Autodesk Fusion 360 part; units mm, degrees
sketch "Sketch1" plane through (0, 0, 0) normal (0, 0, 1) x (1, 0, 0)
  line L0 (50, 50) -> (-50, 50)
  line L1 (-50, 50) -> (-50, -50)
  line L2 (-50, -50) -> (50, -50)
  line L3 (50, -50) -> (50, 50)
  line L4 (50, 50) -> (-50, -50) construction
  line L5 (-50, 50) -> (50, -50) construction
  line L6 (40, -40) -> (-40, -40)
  line L7 (-40, -40) -> (-40, 40)
  line L8 (-40, 40) -> (40, 40)
  line L9 (40, 40) -> (40, -40)
  line L10 (40, -40) -> (-40, 40) construction
  line L11 (-40, -40) -> (40, 40) construction
  dimension "d1" = 100
  dimension "d2" = 100
  dimension "d3" = 80
  dimension "d4" = 80
extrude "Extrude1" add sketch "Sketch1" along normal blind 10
sketch "Sketch2" plane through (0, -40, 0) normal (0, 1, 0) x (-1, 0, 0)
  line L0 (-40, 0) -> (40, 0)
  line L1 (40, 0) -> (40, 10)
  line L2 (40, 10) -> (-40, 10)
  line L3 (-40, 10) -> (-40, 0)
  line L4 (0, 10) -> (0, 0) construction
  line L5 (-40, 5) -> (40, 5) construction
  line L6 (43, 3.5) -> (-43, 3.5)
  line L7 (-43, 3.5) -> (-43, 6.5)
  line L8 (-43, 6.5) -> (43, 6.5)
  line L9 (43, 6.5) -> (43, 3.5)
  line L10 (43, 3.5) -> (-43, 6.5) construction
  line L11 (-43, 3.5) -> (43, 6.5) construction
  point P0 (0, 5)
  dimension "d9" = 86
  dimension "d10" = 3
extrude "Extrude2" cut sketch "Sketch2" along normal blind 85 and the other way blind 5 contours L1 L3 L6 L8
extrude "Extrude3" cut sketch "Sketch2" along normal blind 80 contours L3 L6 L7 L8 | L1 L6 L8 L9
sketch "Sketch3" plane through (0, 0, 10) normal (0, 0, 1) x (-1, 0, 0)
  line L0 (40, -40) -> (-40, -40)
  line L1 (-40, -40) -> (-40, 40)
  line L2 (-40, 40) -> (40, 40)
  line L3 (40, 40) -> (40, -40)
  line L4 (-50, 50) -> (-50, -50)
  line L5 (-50, -50) -> (50, -50)
  line L6 (50, -50) -> (50, 50)
  line L7 (50, 50) -> (-50, 50)
  line L8 (40, -40) -> (40, -50) construction
  line L9 (40, -40) -> (50, -40) construction
  line L10 (45, -40) -> (45, -50) construction
  line L11 (40, -45) -> (50, -45) construction
  circle A0 centre (45, -45) radius 2.5
  circle A1 centre (45, 45) radius 2.5
  dimension "d17" = 5
  dimension "d20" = -90
  dimension "d21" = 90
extrude "Extrude4" cut sketch "Sketch3" against normal blind 3 contours A0 | A1
sketch "Sketch4" plane through (50, 0, 0) normal (1, 0, 0) x (0, 1, 0)
  line L0 (-50, 0) -> (50, 0)
  line L1 (50, 0) -> (50, 10)
  line L2 (50, 10) -> (-50, 10)
  line L3 (-50, 10) -> (-50, 0)
  line L4 (-40, 3.5) -> (-40, 6.5)
  line L5 (-40, 5) -> (-50, 5) construction
  circle A0 centre (-45, 5) radius 2.5
  circle A1 centre (0, 5) radius 2.5
  circle A2 centre (45, 5) radius 2.5
  dimension "d24" = 5
  dimension "d27" = 90
  dimension "d28" = 0
extrude "Extrude5" cut sketch "Sketch4" against normal blind 3 contours A0 | A2
equation "d9 = 80 mm + 6 mm"
equation "d30 = f8e7f7a2-a6e5-415b-bf69-f4a3084041c5"
Source: CAD feature listing. Evaluate the final solid. Frame: model axes, mm. A direction names the side the tool comes from. Give positions to 0.01 mm unless a question says otherwise; leave off trailing zeros. Write each loop counter-clockwise with the first axis right and the second up, starting at its lowest first coordinate (ties: lowest second). Pieces come first, ordered by that corner, then holes. Notation, with made-up numbers: M 39,71 L 52,71 A23 cw 52,96 Z; hole C 47,83.25 d7. An arc over 180 degrees is marked long. Return JSON: item names as keys, results as strings. Group by question number.
1) Cut plane C-C, the plane z = 5. Output: boundary loops of the cut face in (x, y), then the cut area to 3 significant figures.
2) Draft query along X for faces 6 (the face through (-1, -50, 5)), 7 (the face through (-50, 1, 5)), 8 (the face through (47, -45, 5)), 9 (the face through (40, -42, 5)). Return one class per face: released by +X, released by -X, zero draft, split by the parting line, or undercut.
3) Ray query, L1, parallel to Y at x = -45, z = 9; L2, parallel to Y at x = -1, z = 1.75; L3, parallel to Z at x = 1.5, y = -44.5. Return the intervals inside material, ascending.
4) Cut plane A-A, the plane y = -23.5. Output: boundary loops of the cut face in (x, z).
5) Cut plane D-D, the plane x = -45. Output: boundary loops of the cut face in (y, z).
6) Cut plane B-B, the plane x = 15.5. Output: boundary loops of the cut face in (y, z).
7) Set-up query: faces 1 (the face through (-41, -1, 6.5)), 2 (the face through (47, 45, 5)), 3 (the face through (40, 1, 2)), 4 (the face through (-45, 1, 0)), 5 (the face through (-45, 45, 7)). Return all of +Z, -Z, +X, -X, +Y, -Y with unobstructed straight access to the full face (end or side cutting, diameter ignored); none if empty.
Data:
{
 "1": {"outline": "M -50,-50 L 50,-50 L 50,-47.5 L 47,-47.5 L 47,-42.5 L 50,-42.5 L 50,42.5 L 47,42.5 L 47,47.5 L 50,47.5 L 50,50 L -50,50 Z; hole M -43,-40 L -40,-40 L -40,-45 L 40,-45 L 40,-40 L 43,-40 L 43,40 L 40,40 L 40,45 L -40,45 L -40,40 L -43,40 Z", "area": "2,290 mm²"},
 "2": {"face 6": "zero draft", "face 7": "released by -X", "face 8": "released by +X", "face 9": "undercut"},
 "3": {"L1": "y = -50 to -47.5, -42.5 to 42.5, 47.5 to 50", "L2": "y = -50 to -40, 40 to 50", "L3": "z = 0 to 3.5, 6.5 to 10"},
 "4": {"outline": "M -50,0 L -40,0 L -40,3.5 L -43,3.5 L -43,6.5 L -40,6.5 L -40,10 L -50,10 Z; M 40,0 L 50,0 L 50,10 L 40,10 L 40,6.5 L 43,6.5 L 43,3.5 L 40,3.5 Z"},
 "5": {"outline": "M -50,0 L 50,0 L 50,10 L 47.5,10 L 47.5,7 L 42.5,7 L 42.5,10 L -42.5,10 L -42.5,7 L -47.5,7 L -47.5,10 L -50,10 Z"},
 "6": {"outline": "M -50,0 L -40,0 L -40,3.5 L -45,3.5 L -45,6.5 L -40,6.5 L -40,10 L -50,10 Z; M 40,0 L 50,0 L 50,10 L 40,10 L 40,6.5 L 45,6.5 L 45,3.5 L 40,3.5 Z"},
 "7": {"face 1": "none", "face 2": "+X", "face 3": "+Z, -Z", "face 4": "-Z, +X, -X, +Y, -Y", "face 5": "+Z"}
}
